Design review of the part built by this model. Coordinates are the model's own, in mm. A direction names the side the tool comes from. Coordinates: 2 decimals unless noted, no trailing zeros. Loops run counter-clockwise (first coordinate to the right, second up) from the corner with the lowest first, then second, coordinate; pieces in that order, holes last. Notation, with made-up numbers: (2.5, 86.25) - (61.5, 86.25) arc R20 cw to (61.5, 118.25) - close; hole circle Ø5 at (16, 88). An arc over 180 degrees is marked (long way). One line per question, with ' | ' between items.
from build123d import *

# Parameters (mm, degrees)
F0_W     = 45
F0_H     = 45
F1_DEPTH = 2
F2_W     = 22
F2_H     = 22
F2_W_2   = 18
F2_H_2   = 18
F3_DEPTH = 10
F4_W     = 22
F4_H     = 22
F4_W_2   = 2
F4_H_2   = 12
F4_W_3   = 14
F4_H_3   = 2
F4_W_4   = 13
F5_DEPTH = 2
F6_R     = 1.99999
F7_W     = 11
F7_H     = 8
F7_W_2   = 8
F7_H_2   = 11
F8_DEPTH = 12


# Not quite as in the source:
# - a fillet or chamfer is up to 0.001 mm smaller than in the source, because OpenCascade refuses the exact size


with BuildPart() as f1:
    # F0 (on Top) → F1 (new body)
    with BuildSketch(Plane.XY):
        with Locations((22.5, -22.5)):
            Rectangle(F0_W, F0_H)
    extrude(amount=F1_DEPTH)

    # F2 (on face) → F3 (join)
    with BuildSketch(Plane.XY.offset(2)):
        with Locations((34, -34)):
            Rectangle(F2_W, F2_H)
        with Locations((34, -34)):
            Rectangle(F2_W_2, F2_H_2, mode=Mode.SUBTRACT)
    extrude(amount=F3_DEPTH)

    # F4 (on face) → F5 (join)
    with BuildSketch(Plane.XY.offset(12)):
        with Locations((34, -34)):
            Rectangle(F4_W, F4_H)
        Polygon((28, -43), (25, -43), (25, -40), (25, -28), (25, -25), (27, -25), (41, -25), (43, -25), (43, -28), (43, -40), (43, -43), (41, -43), align=None, mode=Mode.SUBTRACT)
        with Locations((26, -34)):
            Rectangle(F4_W_2, F4_H_2)
        with Locations((34, -26)):
            Rectangle(F4_W_3, F4_H_3)
        with Locations((42, -34)):
            Rectangle(F4_W_2, F4_H_2)
        with Locations((34.5, -42)):
            Rectangle(F4_W_4, F4_H_3)
    extrude(amount=F5_DEPTH)

    # F6 (radius 2 in the source; OpenCascade refuses exactly that, so slightly less here)
    f6_edges = [f1.edges().sort_by_distance(p)[0] for p in [
        (25, -34, 12),
        (43, -34, 12),
        (34, -25, 12),
        (34.5, -43, 12),
    ]]
    fillet(f6_edges, radius=F6_R)

    # F7 (on face) → F8 (cut, through all)
    with BuildSketch(Plane.XY.offset(14)):
        with Locations((43.5, -34)):
            Rectangle(F7_W, F7_H)
        with Locations((34, -43.5)):
            Rectangle(F7_W_2, F7_H_2)
        with Locations((34, -34)):
            Rectangle(F7_W_2, F7_H)
        with Locations((24.5, -34)):
            Rectangle(F7_W, F7_H)
        with Locations((34, -24.5)):
            Rectangle(F7_W_2, F7_H_2)
    extrude(amount=-F8_DEPTH, mode=Mode.SUBTRACT)


solid = f1.part
Q1. Take a section at D-D (x = 31.5). Give the boundary of the cut face in (y, z), plus the area to 3 significant figures.
Returned:
outline: (-45, 0) - (0, 0) - (0, 2) - (-45, 2) - close | area: 90.0 mm²
Q2. Tool access review of faces 1 (the flat face through (0, -23, 1)), 2 (the flat face through (38, -43.5, 9.4)), 3 (the cylindrical face through (39.52, -25.6, 11.43)), 4 (the flat face through (41, -26, 13)), 5 (the flat face through (23, -42, 8)): name each direction out of +Z, -Z, +X, -X, +Y, -Y from which nothing blocks a thin tool from reaching the whole face with its end or side.
Returned:
face 1: +Z, -Z, -X, +Y, -Y | face 2: +Z, +Y, -Y | face 3: none | face 4: +Z | face 5: +Z, -X, +Y, -Y
Q3. Take a section at A-A (z = 7.75). Give the boundary of the cut face in (x, y).
Returned:
outline: (23, -45) - (30, -45) - (30, -43) - (25, -43) - (25, -38) - (23, -38) - close; (23, -30) - (25, -30) - (25, -25) - (30, -25) - (30, -23) - (23, -23) - close; (38, -45) - (45, -45) - (45, -38) - (43, -38) - (43, -43) - (38, -43) - close; (38, -25) - (43, -25) - (43, -30) - (45, -30) - (45, -23) - (38, -23) - close
Q4. Take a section at B-B (x = 42). Give the boundary of the cut face in (y, z).
Returned:
outline: (-45, 0) - (0, 0) - (0, 2) - (-23, 2) - (-23, 14) - (-25, 14) - (-25, 2) - (-43, 2) - (-43, 14) - (-45, 14) - close; (-40, 11.73) - (-38, 11.73) - (-38, 14) - (-40, 14) - close; (-30, 11.73) - (-28, 11.73) - (-28, 14) - (-30, 14) - close
Q5. For pin 1 (8 mm diameter, centred on x = 28, y = -8, fed in from +Z); pin 2 (4 mm diameter, centred on x = 40, z = 6.5, fed in from +Y); pin 3 (6 mm diameter, centred on y = -36.5, z = 10.5, fed in from -X); pin 4 (2 mm diameter, centred on y = -36.5, z = 9.5, fed in from -X), all flat-tipped, find the tip position at first contact; note any pin that passes through.
Returned:
pin 1: stops at z = 2 | pin 2: stops at y = -23 | pin 3: stops at x = 23 | pin 4: passes through
Q6. To check wall thickness, follow line 1 along X through (y, z) = (-28.5, 5.5); line 2 along Y through (x, z) = (43.5, 7.5); line 3 along Y through (x, z) = (42, 8.5). State the ranges of each line that lie inside material, in increasing order.
Returned:
line 1: x = 23 to 25, 43 to 45 | line 2: y = -45 to -38, -30 to -23 | line 3: y = -45 to -43, -25 to -23
Q7. Draft analysis for pull direction X (two halves, no side actions). For faces 6 (the flat face through (27.2, -25.7, 14)), 7 (the flat face through (23, -27, 8)), 8 (the flat face through (27, -39, 13)), 9 (the flat face through (28, -27, 13)), state which applies: +X half, -X half, draft (parallel to the pull), parting line (faces both ways), or undercut.
Returned:
face 6: draft | face 7: -X half | face 8: undercut | face 9: undercut
Q8. Take a section at C-C (y = -36). Give the boundary of the cut face in (x, z), plus the area to 3 significant figures.
Returned:
outline: (0, 0) - (45, 0) - (45, 2) - (0, 2) - close | area: 90.0 mm²
